The listing builds one solid part. Answer for the finished solid, in the listing's coordinates (mm). Round coordinates to 2 decimals unless told otherwise and drop trailing zeros. Loops run counter-clockwise (first coordinate to the right, second up) from the corner with the lowest first, then second, coordinate; pieces in that order, holes last. Notation, with made-up numbers: (36, -37) -> (94, -37) arc R36 cw to (94, 1) -> close; hole circle Ø5 at (74, 6.25). An arc over 180 degrees is marked (long way). Write each question's results on one line, items separated by ' | '. Start each with the question number.
from build123d import *

# Parameters (mm, degrees)
F1_DEPTH    = 10
F2_T1_DEPTH = 61.905591591


# Not quite as in the source:
# - a fillet or chamfer that OpenCascade refuses, or shapes differently, is made with other operations: its cross-section is extruded or revolved along the edge and cut away or added


with BuildPart() as f1:
    # F0 (on Front) → F1 (new body)
    with BuildSketch(Plane.XZ):
        Polygon((-34.8533578217, 10), (-34.8533578217, 0), (25.1466421783, 0), (25.1466421783, 20), (-34.8533578217, 20), align=None)
        with BuildLine():
            ThreePointArc((-19.8533578217, 10), (-24.8533578217, 5), (-29.8533578217, 10))
            ThreePointArc((-29.8533578217, 10), (-24.8533578217, 15), (-19.8533578217, 10))
        make_face(mode=Mode.SUBTRACT)
    extrude(amount=F1_DEPTH)

    # F2: fillet of radius 10.3811183182 on 2 edges, made by hand

    # F2_s2 → F2_t1 (cut)
    with BuildSketch(Plane.XZ.offset(-25.9527957955)):
        with BuildLine():
            ThreePointArc((-24.4722395035, 20), (-31.8127986626, 16.9594408409), (-34.8533578217, 9.6188816818))
            Line((-34.8533578217, 9.6188816818), (-34.8533578217, 20))
            Line((-34.8533578217, 20), (-24.4722395035, 20))
        make_face()
        with BuildLine():
            ThreePointArc((-24.4722395035, 0), (-31.8127986626, 3.0405591591), (-34.8533578217, 10.3811183182))
            Line((-34.8533578217, 10.3811183182), (-34.8533578217, 0))
            Line((-34.8533578217, 0), (-24.4722395035, 0))
        make_face()
    extrude(amount=F2_T1_DEPTH, mode=Mode.SUBTRACT)


solid = f1.part
Item 1: The part is cut by section A-A, the plane y = -6.5. Give the vertices of the cut face in (x, z).
Item 2: Straight lines are drawn through the part: L1, parallel to X at y = -1, z = 9.5; L2, parallel to X at y = -3, z = 6.25; L3, parallel to X at y = -9.25, z = 3.25. For each, find the intervals that lie inside material, in ascending order. Write a range as [from, to].
Item 3: Determine the mould class of faces 1 (the cylindrical face through (-19.86, -4.93, 10.22)), 2 (the flat face through (25.147, -5, 10)), 3 (the flat face through (-5, -10, 10)) for opening direction X: +X half, -X half, draft (parallel to the pull), parting line (faces both ways), or undercut.
Item 4: The part is cut by section B-B, the plane z = 6.5. Give the vertices of the cut face in (x, y), plus the area to 3 significant figures.
Item 5: This flat-tipped pin is pushed along its axis until it touches: pin 1 Ø9 at (x, z) = (-24.85, 10) entering from -Y. Where does it stop, or does it pass through?
Item 6: The part is cut by section C-C, the plane x = -21.5. Give the vertices of the cut face in (y, z).
Item 7: The part is cut by section D-D, the plane z = 16. Give the vertices of the cut face in (x, y), plus the area to 3 significant figures.
Report:
1) outline: (-34.85, 10) arc R10.38 ccw to (-24.47, 0) -> (25.15, 0) -> (25.15, 20) -> (-24.47, 20) arc R10.38 ccw to start; hole circle Ø10 at (-24.85, 10)
2) L1: x = [-34.82, -29.83], [-19.88, 25.15] | L2: x = [-34, -28.16], [-21.55, 25.15] | L3: x = [-32.02, 25.15]
3) face 1: undercut | face 2: +X half | face 3: draft
4) outline: (-34.1, -10) -> (-28.42, -10) -> (-28.42, 0) -> (-34.1, 0) -> close; (-21.28, -10) -> (25.15, -10) -> (25.15, 0) -> (-21.28, 0) -> close | area: 521 mm2
5) pin 1: passes through
6) outline: (-10, 0) -> (0, 0) -> (0, 6.29) -> (-10, 6.29) -> close; (-10, 13.71) -> (0, 13.71) -> (0, 20) -> (-10, 20) -> close
7) outline: (-32.66, -10) -> (25.15, -10) -> (25.15, 0) -> (-32.66, 0) -> close | area: 578 mm2
